The listing builds one solid part. Answer for the finished solid, in the listing's coordinates (mm). Face numbers are marked on the shaded views. A direction names the side the tool comes from. Give positions to 0.01 mm unless a question says otherwise; leave off trailing zeros. Write each loop counter-clockwise with the first axis right and the second up, starting at its lowest first coordinate (ties: lowest second). Pieces come first, ordered by that corner, then holes. Notation, with made-up numbers: M 32,31.25 L 60,31.25 A22 cw 60,66.25 Z; hole C -21.75,12.5 d7. An arc over 180 degrees is marked long. Answer as a JSON object with one key per item and string values.
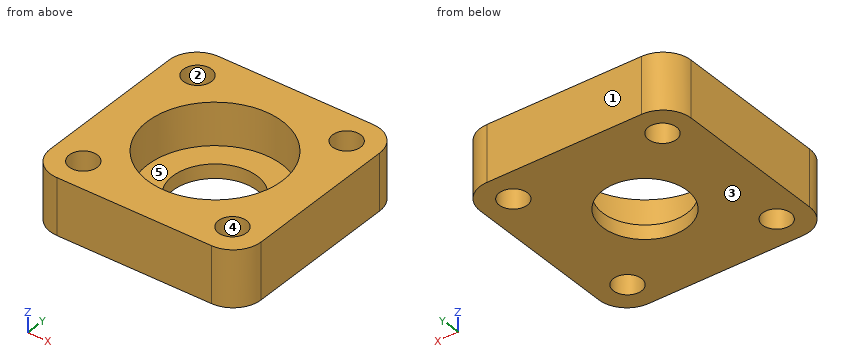
```python
from build123d import *

# Parameters (mm, degrees)
SKETCH1_W           = 30
SKETCH1_H           = 30
SKETCH1_R           = 2
BOSS_EXTRUDE1_DEPTH = 8
SKETCH2_R           = 9.6
CUT_EXTRUDE1_DEPTH  = 6
SKETCH3_R           = 6
CUT_EXTRUDE2_DEPTH  = 7
FILLET1_R           = 4


with BuildPart() as part:
    # Sketch1 → Boss-Extrude1 (new body)
    with BuildSketch(Plane.XY):
        with Locations((15, 15)):
            Rectangle(SKETCH1_W, SKETCH1_H)
        with Locations((25.606601718, 25.606601718)):
            Circle(SKETCH1_R, mode=Mode.SUBTRACT)
        with Locations((25.606601718, 4.393398282)):
            Circle(SKETCH1_R, mode=Mode.SUBTRACT)
        with Locations((4.393398282, 4.393398282)):
            Circle(SKETCH1_R, mode=Mode.SUBTRACT)
        with Locations((4.393398282, 25.606601718)):
            Circle(SKETCH1_R, mode=Mode.SUBTRACT)
    extrude(amount=BOSS_EXTRUDE1_DEPTH)

    # Sketch2 → Cut-Extrude1 (cut)
    with BuildSketch(Plane.XY.offset(8)):
        with Locations((15, 15)):
            Circle(SKETCH2_R)
    extrude(amount=-CUT_EXTRUDE1_DEPTH, mode=Mode.SUBTRACT)

    # Sketch3 → Cut-Extrude2 (cut)
    with BuildSketch(Plane.XY.offset(2)):
        with Locations((15, 15)):
            Circle(SKETCH3_R)
    extrude(amount=-CUT_EXTRUDE2_DEPTH, mode=Mode.SUBTRACT)

    # Fillet1
    fillet1_edges = [part.edges().sort_by_distance(p)[0] for p in [
        (0, 30, 4),
        (30, 30, 4),
        (30, 0, 4),
        (0, 0, 4),
    ]]
    fillet(fillet1_edges, radius=FILLET1_R)


solid = part.part
```
1. A cutting plane is placed at A-A, the plane x = 15. Give the vertices of the cut face in (y, z), plus the area to 3 significant figures.
Verdict:
{"outline": "M 0,0 L 9,0 L 9,2 L 5.4,2 L 5.4,8 L 0,8 Z; M 21,0 L 30,0 L 30,8 L 24.6,8 L 24.6,2 L 21,2 Z", "area": "101 mm2"}
2. A cutting plane is placed at C-C, the plane z = 1.5. Give the vertices of the cut face in (x, y), plus the area to 3 significant figures.
Verdict:
{"outline": "M 0,4 A4 ccw 4,0 L 26,0 A4 ccw 30,4 L 30,26 A4 ccw 26,30 L 4,30 A4 ccw 0,26 Z; hole C 4.39,4.39 d4; hole C 4.39,25.61 d4; hole C 15,15 d12; hole C 25.61,4.39 d4; hole C 25.61,25.61 d4", "area": "723 mm2"}
3. For the marked faces 4 and 5, determine the directions among +Z, -Z, +X, -X, +Y, -Y from which every point of the face is accessible in a straight line to the end or side of a thin tool.
Verdict:
{"face 4": "+Z, -Z", "face 5": "+Z"}
4. A flat-ended cylindrical pin translates along its axis: pin 1 (9.5 mm diameter, centred on x = 17, y = 11.5, fed in from +Z). Find the tip coordinate at first contact, or state that the pin passes through.
Verdict:
{"pin 1": "stops at z = 2"}
5. The mould has two halves that part along Y. Classify the marked faces 1, 2 and 3: released by +Y, released by -Y, zero draft, split by the parting line, or undercut.
Verdict:
{"face 1": "released by +Y", "face 2": "undercut", "face 3": "zero draft"}
6. Consider line 1 along Y through (x, z) = (25.75, 6.5); line 2 along Y through (x, z) = (3.5, 7.25); line 3 along Y through (x, z) = (15, 0.8). Determine where each line is inside the solid, lowest interval first.
Verdict:
{"line 1": "y = 0 to 2.4, 6.39 to 23.61, 27.6 to 30", "line 2": "y = 0.03 to 2.6, 6.18 to 23.82, 27.4 to 29.97", "line 3": "y = 0 to 9, 21 to 30"}
7. A cutting plane is placed at D-D, the plane x = 7.75. Give the vertices of the cut face in (y, z), plus the area to 3 significant figures.
Verdict:
{"outline": "M 0,0 L 30,0 L 30,8 L 21.29,8 L 21.29,2 L 8.71,2 L 8.71,8 L 0,8 Z", "area": "164 mm2"}
